Model file for the job. Use its own axes, mm. A direction names the side the tool comes from. Coordinates: 2 decimals unless noted, no trailing zeros. Order: outer loops, then holes, each group sorted by start corner. A loop starts at its lowest first (then second) coordinate and runs counter-clockwise, first axis right, second up.
from build123d import *

# Parameters (mm, degrees)
F0_W           = 44.45
F0_H           = 57.15
F1_DEPTH       = 38.1
F4_D           = 26.19375
F6_D           = 8.73125
F6_CBORE_D     = 13.4874
F6_CBORE_DEPTH = 9.525


with BuildPart() as f1:
    # F0 (on Top) → F1 (new body)
    with BuildSketch(Plane.XY):
        Rectangle(F0_W, F0_H)
    extrude(amount=F1_DEPTH)

    # F4 (through all)
    with Locations(Plane.XY.offset(38.1)):
        with Locations((0, 0)):
            Hole(F4_D / 2)

    # F6 (through all)
    with Locations(Plane.XY.offset(38.1)):
        with Locations((-14.605, 20.955), (14.605, 20.955), (14.605, -20.955), (-14.605, -20.955)):
            CounterBoreHole(F6_D / 2, F6_CBORE_D / 2, F6_CBORE_DEPTH)


solid = f1.part
Q1. Drop a flat-ended pin along its axis: P1, Ø11, axis at x = -14.605, y = -20.955, coming from the +Z side (3 decimals). Give the stop position or say it passes through.
Established:
P1: stops at z = 28.575
Q2. Cut at B-B, the plane y = 0. List the corners of the cut face in (x, z) (3 decimals), plus the area to 3 significant figures.
Established:
outline: (-22.225, 0) - (-13.097, 0) - (-13.097, 38.1) - (-22.225, 38.1) - close; (13.097, 0) - (22.225, 0) - (22.225, 38.1) - (13.097, 38.1) - close
area: 696 mm2
Q3. Mould opens along X. For faces 3 (the face through (-22.225, 0, 19)), 4 (the face through (22.225, 0, 19)), 5 (the face through (0, 28.575, 19)), 6 (the face through (-15.48, 27.64, 33.4)) say: pulls with the +X half, pulls with the -X half, needs draft (parallel to the pull), parting line crosses it, or undercut.
Established:
face 3: pulls with the -X half
face 4: pulls with the +X half
face 5: needs draft
face 6: undercut
Q4. Probe line 1 (Y direction, x = -9, z = 32.5) (3 decimals); line 2 (Y direction, x = 0, z = 17) (3 decimals); line 3 (Y direction, x = -18, z = 12) (3 decimals). List the from-to ranges inside material, lowest first.
Established:
line 1: y = -28.575 to -24.705, -17.205 to -9.515, 9.515 to 17.205, 24.705 to 28.575
line 2: y = -28.575 to -13.097, 13.097 to 28.575
line 3: y = -28.575 to -23.7, -18.21 to 18.21, 23.7 to 28.575
Q5. Which spindle directions (+Z, -Z, +X, -X, +Y, -Y) get a long thin tool onto all of the face, cutting with end or side? Do faces 1 (the face through (16, -25.4, 28.575)), 2 (the face through (-10.244, 21.147, 14.087)). Say none if no direction does.
Established:
face 1: +Z
face 2: +Z, -Z
Q6. Cut at C-C, the plane z = 7. List the corners of the cut face in (x, y) (3 decimals), plus the area to 3 significant figures.
Established:
outline: (-22.225, -28.575) - (22.225, -28.575) - (22.225, 28.575) - (-22.225, 28.575) - close; hole circle Ø8.731 at (-14.605, -20.955); hole circle Ø8.731 at (-14.605, 20.955); hole circle Ø26.194 at (0, 0); hole circle Ø8.731 at (14.605, -20.955); hole circle Ø8.731 at (14.605, 20.955)
area: 1,760 mm2
Q7. Cut at A-A, the plane x = 0. List the corners of the cut face in (y, z) (3 decimals).
Established:
outline: (-28.575, 0) - (-13.097, 0) - (-13.097, 38.1) - (-28.575, 38.1) - close; (13.097, 0) - (28.575, 0) - (28.575, 38.1) - (13.097, 38.1) - close
Q8. Cut at D-D, the plane y = 20. List the corners of the cut face in (x, z) (3 decimals), plus the area to 3 significant figures.
Established:
outline: (-22.225, 0) - (-18.865, 0) - (-18.865, 28.575) - (-21.281, 28.575) - (-21.281, 38.1) - (-22.225, 38.1) - close; (-10.345, 0) - (10.345, 0) - (10.345, 28.575) - (7.929, 28.575) - (7.929, 38.1) - (-7.929, 38.1) - (-7.929, 28.575) - (-10.345, 28.575) - close; (18.865, 0) - (22.225, 0) - (22.225, 38.1) - (21.281, 38.1) - (21.281, 28.575) - (18.865, 28.575) - close
area: 952 mm2
